Input: dimensioned drawing with shaded views. Units: mm. Origin: part minimum x, y, z. A direction names the side the tool comes from. Give positions to 0.01 mm unless a question says otherwise; leave off trailing zeros. Write each loop counter-clockwise with the first axis right and the second up, starting at its lowest first coordinate (ties: lowest second). Pieces come first, ordered by that corner, then holes. Notation, with made-up numbers: M -38.75,-17.5 L 11.25,-17.5 A14 ccw 11.25,7.5 Z; hole C 34,72 d1. An arc over 180 degrees is marked long. Answer as a JSON object with one key per item and string values.
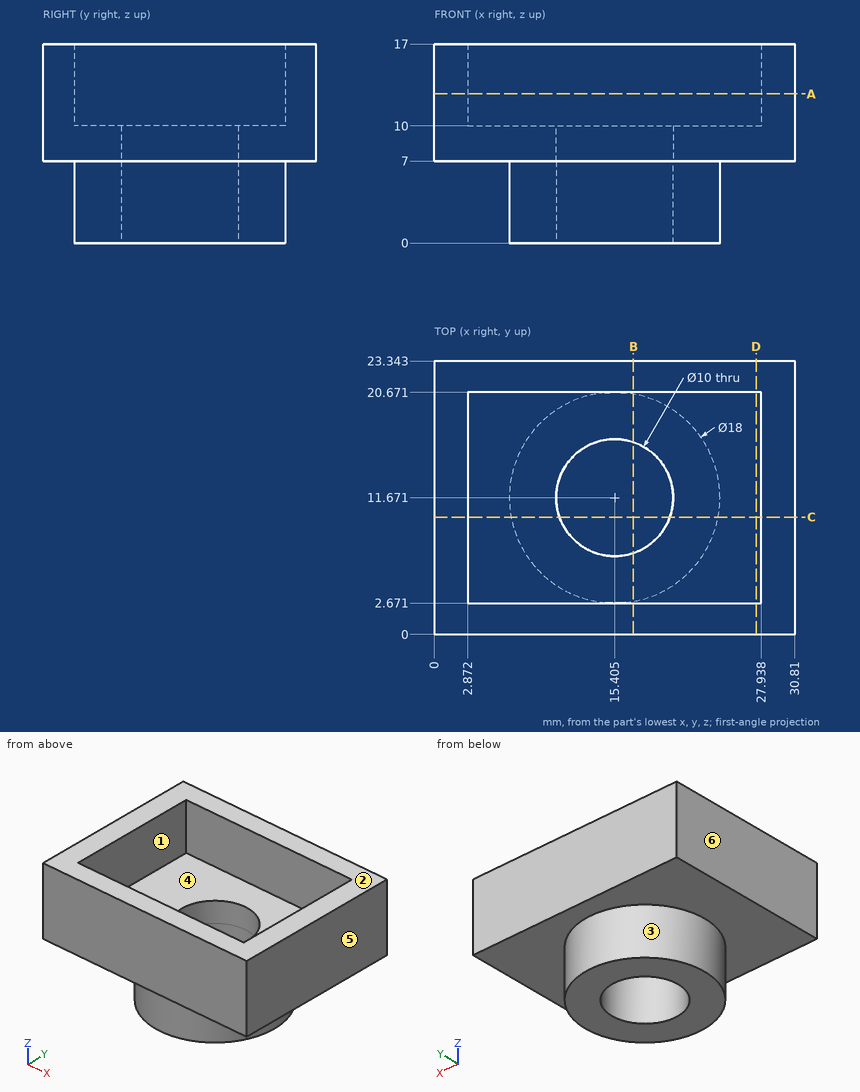
1) Set-up query: the marked faces 1, 2 and 3. Return all of +Z, -Z, +X, -X, +Y, -Y with unobstructed straight access to the full face (end or side cutting, diameter ignored); none if empty.
Geometry check:
{"face 1": "+Z", "face 2": "+Z, +X, -X, +Y, -Y", "face 3": "-Z"}
2) Cut plane A-A on z = 12.75. Return loops of the section in (x, y), and give its area (3 significant figures).
Geometry check:
{"outline": "M 0,0 L 30.81,0 L 30.81,23.34 L 0,23.34 Z; hole M 2.87,2.67 L 27.94,2.67 L 27.94,20.67 L 2.87,20.67 Z", "area": "268 mm2"}
3) Line query: line 1 (Y direction, x = 10, z = 14.75); line 2 (X direction, y = 11.75, z = 14); line 3 (Z direction, x = 17, y = 3). Output: solid intervals per line, ascending. Write a range as from..to.
Geometry check:
{"line 1": "y = 0..2.67, 20.67..23.34", "line 2": "x = 0..2.87, 27.94..30.81", "line 3": "z = 0..10"}
4) Cut plane B-B on x = 17. Return loops of the section in (y, z).
Geometry check:
{"outline": "M 0,7 L 2.81,7 L 2.81,0 L 6.93,0 L 6.93,10 L 2.67,10 L 2.67,17 L 0,17 Z; M 16.41,0 L 20.53,0 L 20.53,7 L 23.34,7 L 23.34,17 L 20.67,17 L 20.67,10 L 16.41,10 Z"}
5) Cut plane C-C on y = 10. Return loops of the section in (x, z).
Geometry check:
{"outline": "M 0,7 L 6.56,7 L 6.56,0 L 10.69,0 L 10.69,10 L 2.87,10 L 2.87,17 L 0,17 Z; M 20.12,0 L 24.25,0 L 24.25,7 L 30.81,7 L 30.81,17 L 27.94,17 L 27.94,10 L 20.12,10 Z"}
6) Cut plane D-D on x = 27.5. Return loops of the section in (y, z).
Geometry check:
{"outline": "M 0,7 L 23.34,7 L 23.34,17 L 20.67,17 L 20.67,10 L 2.67,10 L 2.67,17 L 0,17 Z"}
7) Contact query for flat-ended pins moving along their axis: P1, Ø1.5, axis at x = 25.5, y = 9, coming from the -Z side; P2, Ø5, axis at x = 5.5, y = 17, coming from the +Z side. Output: stop coordinate, or through.
Geometry check:
{"P1": "stops at z = 7", "P2": "stops at z = 10"}
8) Pull-direction query (X, two-part tool) for the marked faces 4, 5 and 6; classes: pulls with the +X half, pulls with the -X half, needs draft (parallel to the pull), parting line crosses it, or undercut.
Geometry check:
{"face 4": "undercut", "face 5": "pulls with the +X half", "face 6": "pulls with the -X half"}
